```python
from build123d import *

# Parameters (mm, degrees)
SKETCH_1_W                         = 125
SKETCH_1_H                         = 42
SM_BASE_FLANGE_490_DEPTH           = 2
SM_EDGE_FLANGE_503_STRIP_W         = 9.4732
SM_EDGE_FLANGE_503_STRIP_H         = 2
SM_EDGE_FLANGE_503_STRIP_CUT_DEPTH = 42
SM_EDGE_FLANGE_503_DEPTH           = 42
SM_EDGE_FLANGE_662_STRIP_W         = 9.4732
SM_EDGE_FLANGE_662_STRIP_H         = 2
SM_EDGE_FLANGE_662_STRIP_CUT_DEPTH = 42
SM_EDGE_FLANGE_662_DEPTH           = 42
FILLET_810_R                       = 3
EXTRUDE_START                      = -129
EXTRUDE_1524_OUTLINE_R             = 1.5
EXTRUDE_1524_OUTLINE_R_2           = 12.5
EXTRUDE_1524_DEPTH                 = 129
EXTRUDE_START_2                    = -2
EXTRUDE_2057_OUTLINE_W             = 10
EXTRUDE_2057_OUTLINE_H             = 20
EXTRUDE_2057_DEPTH                 = 2
HOLE_WIZARD_M2_D                   = 2


# Read off the part's stored shape, not the designer's step: 电机螺丝孔, 车架接口
# Sheet-metal steps are written as plain solids
with BuildPart() as part:
    # Sketch 1 → Sm Base Flange 490 (new body)
    with BuildSketch(Plane(origin=(0, 0, 0), x_dir=(1, 0, 0), z_dir=(0, 1, 0))):
        with Locations((6.143518865, -7.014413587)):
            Rectangle(SKETCH_1_W, SKETCH_1_H)
    extrude(amount=-SM_BASE_FLANGE_490_DEPTH)

    # Sm Edge Flange 503 strip (across the edge) → Sm Edge Flange 503 strip cut (cut)
    with BuildSketch(Plane(origin=(-56.356481135, -2, 28.014413587), x_dir=(1, 0, 0), z_dir=(0, 0, -1))):
        with Locations((-4, -1)):
            Rectangle(SM_EDGE_FLANGE_503_STRIP_W, SM_EDGE_FLANGE_503_STRIP_H)
    extrude(amount=SM_EDGE_FLANGE_503_STRIP_CUT_DEPTH, mode=Mode.SUBTRACT)

    # Sm Edge Flange 503 section (across the edge) → Sm Edge Flange 503 (add)
    with BuildSketch(Plane(origin=(-56.356481135, -2, 28.014413587), x_dir=(1, 0, 0), z_dir=(0, 0, -1))):
        with BuildLine():
            Line((-2, 0.7366), (-2, 42))
            Line((-2, 42), (0, 42))
            Line((0, 42), (0, 0.7366))
            ThreePointArc((0, 0.7366), (0.215745145, 0.215745145), (0.7366, 0))
            Line((0.7366, 0), (0.7366, -2))
            ThreePointArc((0.7366, -2), (-1.198468417, -1.198468417), (-2, 0.7366))
        make_face()
    extrude(amount=SM_EDGE_FLANGE_503_DEPTH)

    # Sm Edge Flange 662 strip (across the edge) → Sm Edge Flange 662 strip cut (cut)
    with BuildSketch(Plane(origin=(68.643518865, -2, -13.985586413), x_dir=(-1, 0, 0), z_dir=(0, 0, 1))):
        with Locations((-4, -1)):
            Rectangle(SM_EDGE_FLANGE_662_STRIP_W, SM_EDGE_FLANGE_662_STRIP_H)
    extrude(amount=SM_EDGE_FLANGE_662_STRIP_CUT_DEPTH, mode=Mode.SUBTRACT)

    # Sm Edge Flange 662 section (across the edge) → Sm Edge Flange 662 (add)
    with BuildSketch(Plane(origin=(68.643518865, -2, -13.985586413), x_dir=(-1, 0, 0), z_dir=(0, 0, 1))):
        with BuildLine():
            Line((-2, 0.7366), (-2, 42))
            Line((-2, 42), (0, 42))
            Line((0, 42), (0, 0.7366))
            ThreePointArc((0, 0.7366), (0.215745145, 0.215745145), (0.7366, 0))
            Line((0.7366, 0), (0.7366, -2))
            ThreePointArc((0.7366, -2), (-1.198468417, -1.198468417), (-2, 0.7366))
        make_face()
    extrude(amount=SM_EDGE_FLANGE_662_DEPTH)

    # Fillet 810
    fillet_810_edges = [part.edges().sort_by_distance(p)[0] for p in [
        (-57.356481135, -44, 28.014413587),
        (-57.356481135, -44, -13.985586413),
        (69.643518865, -44, -13.985586413),
        (69.643518865, -44, 28.014413587),
    ]]
    fillet(fillet_810_edges, radius=FILLET_810_R)

    # Extrude 1524 outline → Extrude 1524 (cut)
    with BuildSketch(Plane.ZY.offset(58.356481135).offset(EXTRUDE_START)):
        with Locations((-8.485586413, -7.5)):
            Circle(EXTRUDE_1524_OUTLINE_R)
        with Locations((22.514413587, -7.5)):
            Circle(EXTRUDE_1524_OUTLINE_R)
        with Locations((22.514413587, -38.5)):
            Circle(EXTRUDE_1524_OUTLINE_R)
        with Locations((-8.485586413, -38.5)):
            Circle(EXTRUDE_1524_OUTLINE_R)
        with Locations((7.014413587, -23.7366)):
            Circle(EXTRUDE_1524_OUTLINE_R_2)
    extrude(amount=EXTRUDE_1524_DEPTH, mode=Mode.SUBTRACT)

    # Extrude 2057 outline → Extrude 2057 (cut)
    with BuildSketch(Plane(origin=(0, 0, 0), x_dir=(1, 0, 0), z_dir=(0, 1, 0)).offset(EXTRUDE_START_2)):
        with Locations((47.906918865, -7.014413587)):
            Rectangle(EXTRUDE_2057_OUTLINE_W, EXTRUDE_2057_OUTLINE_H)
        with Locations((-35.619881135, -7.014413587)):
            Rectangle(EXTRUDE_2057_OUTLINE_W, EXTRUDE_2057_OUTLINE_H)
    extrude(amount=EXTRUDE_2057_DEPTH, mode=Mode.SUBTRACT)

    # M2螺纹孔 (through all)
    with Locations(Plane(origin=(0, 0, 0), x_dir=(1, 0, 0), z_dir=(0, 1, 0))):
        with Locations((-29.854881135, 10.985586413), (42.141918865, 10.985586413), (42.141918865, -25.014413587), (-29.854881135, -25.014413587), (-36.354881135, 10.985586413), (48.641918865, 10.985586413), (48.641918865, -25.014413587), (-36.354881135, -25.014413587)):
            Hole(HOLE_WIZARD_M2_D / 2)


solid = part.part
```
Work out the finished part from the listing and answer in its coordinate system (mm). A direction names the side the tool comes from. Give positions to 0.01 mm unless a question says otherwise; leave off trailing zeros. Order: outer loops, then holes, each group sorted by start corner. A loop starts at its lowest first (then second) coordinate and runs counter-clockwise, first axis right, second up.
1. Section B-B, the plane z = 11 is taken. Determine the outline of the cut face in (x, y), and give its area (3 significant figures).
Result sheet:
outline: (-58.36, -44) - (-56.36, -44) - (-56.36, -35.58) - (-58.36, -35.58) - close; (-58.36, -11.89) - (-56.36, -11.89) - (-56.36, -2.74) arc R0.74 cw to (-55.62, -2) - (-40.62, -2) - (-40.62, 0) - (-55.62, 0) arc R2.74 ccw to (-58.36, -2.74) - close; (-30.62, -2) - (42.91, -2) - (42.91, 0) - (-30.62, 0) - close; (52.91, -2) - (67.91, -2) arc R0.74 cw to (68.64, -2.74) - (68.64, -11.89) - (70.64, -11.89) - (70.64, -2.74) arc R2.74 ccw to (67.91, 0) - (52.91, 0) - close; (68.64, -44) - (70.64, -44) - (70.64, -35.58) - (68.64, -35.58) - close
area: 288 mm2
2. Section C-C, the plane y = -15 is taken. Determine the outline of the cut face in (x, z), and give its area (3 significant figures).
Result sheet:
outline: (-58.36, -13.99) - (-56.36, -13.99) - (-56.36, -1.93) - (-58.36, -1.93) - close; (-58.36, 15.95) - (-56.36, 15.95) - (-56.36, 28.01) - (-58.36, 28.01) - close; (68.64, -13.99) - (70.64, -13.99) - (70.64, -1.93) - (68.64, -1.93) - close; (68.64, 15.95) - (70.64, 15.95) - (70.64, 28.01) - (68.64, 28.01) - close
area: 96.5 mm2
3. Section D-D, the plane x = -8 is taken. Determine the outline of the cut face in (y, z).
Result sheet:
outline: (-2, -13.99) - (0, -13.99) - (0, 28.01) - (-2, 28.01) - close
4. Straight lines are drawn through the part: L1, parallel to Z at x = 69.5, y = -38.5; L2, parallel to X at y = -42, z = 0; L3, parallel to Y at x = 37, z = 18.5. For each, find the intervals that lie inside material, in ascending order.
Result sheet:
L1: z = -13.99 to -9.99, -6.99 to 21.01, 24.01 to 28.01
L2: x = -58.36 to -56.36, 68.64 to 70.64
L3: y = -2 to 0
5. Section A-A, the plane y = -7.5 is taken. Determine the outline of the cut face in (x, z), and give its area (3 significant figures).
Result sheet:
outline: (-58.36, -13.99) - (-56.36, -13.99) - (-56.36, -9.99) - (-58.36, -9.99) - close; (-58.36, -6.99) - (-56.36, -6.99) - (-56.36, 21.01) - (-58.36, 21.01) - close; (-58.36, 24.01) - (-56.36, 24.01) - (-56.36, 28.01) - (-58.36, 28.01) - close; (68.64, -13.99) - (70.64, -13.99) - (70.64, -9.99) - (68.64, -9.99) - close; (68.64, -6.99) - (70.64, -6.99) - (70.64, 21.01) - (68.64, 21.01) - close; (68.64, 24.01) - (70.64, 24.01) - (70.64, 28.01) - (68.64, 28.01) - close
area: 144 mm2
6. The mould has two halves that part along Y. Classify faces 3 (the cylindrical face through (69.66, -8.41, 21.32)), 4 (the flat face through (68.644, -33, -3)), 5 (the cylindrical face through (-57.34, -43.1, -13.13)), 6 (the cylindrical face through (-57.34, -39.83, -7.79)): released by +Y, released by -Y, zero draft, split by the parting line, or undercut.
Result sheet:
face 3: undercut
face 4: zero draft
face 5: released by -Y
face 6: undercut
7. Each of these flat-tipped pins is pushed along its axis until it touches: P1, Ø2.5, axis at x = 48.64, z = -10.99, coming from the -Y side; P2, Ø1.8, axis at y = -7.5, z = -8.49, coming from the -X side; P3, Ø0.6, axis at y = -0.5, z = 5, coming from the -X side. Where does it stop, or does it pass through?
Result sheet:
P1: stops at y = -2
P2: passes through
P3: stops at x = -57.55
8. For faces 1 (the flat face through (-56.356, -33, -2)), 2 (the cylindrical face through (69.63, -43.145, -13.083)), determine the directions among +Z, -Z, +X, -X, +Y, -Y from which every point of the face is accessible in a straight line to the end or side of a thin tool.
Result sheet:
face 1: +Z, -Z, -Y
face 2: -Z, +X, -X, -Y
